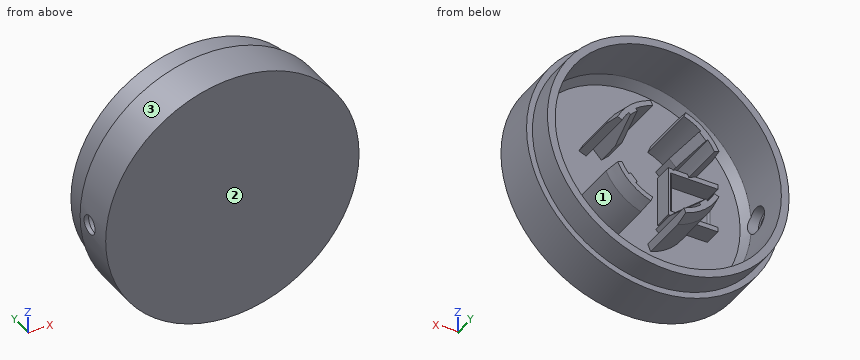
from build123d import *
from OCP.BRepFilletAPI import BRepFilletAPI_MakeChamfer

# Parameters (mm, degrees)
EXTRUDE_1_DEPTH     = 7
OTHER_START         = -47.7
OTHER_1_OUTLINE_R   = 5.1
OTHER_1_DEPTH       = 35.8
OTHER_START_2       = -30.461492928
OTHER_1_2_DEPTH     = 18.561492928
OTHER_START_3       = -51
OTHER_1_3_OUTLINE_R = 3.65
OTHER_1_3_DEPTH     = 3.3
OTHER_START_4       = 2
OTHER_1_4_DEPTH     = 1
OTHER_START_5       = 2.8
OTHER_1_5_DEPTH     = 7.2
OTHER_START_6       = -3
OTHER_1_6_DEPTH     = 0.709959236
EXTRUDE_2_DEPTH     = 24
EXTRUDE_2_2_DEPTH   = 24
EXTRUDE_2_3_DEPTH   = 24
EXTRUDE_2_4_DEPTH   = 24
CHAMFER_1_SIZE      = 6
CHAMFER_1_SIZE2     = 1.057961884
CHAMFER_2_SIZE      = 6
CHAMFER_2_SIZE2     = 1.057961884
CHAMFER_3_SIZE      = 6
CHAMFER_3_SIZE2     = 1.057961884
CHAMFER_4_SIZE      = 6
CHAMFER_4_SIZE2     = 1.057961884
CHAMFER_5_SIZE      = 1.1
EXTRUDE_3_DEPTH     = 24
CHAMFER_6_SIZE      = 15
CHAMFER_6_SIZE2     = 4.019237886


with BuildPart() as part:
    # Sketch 1 → Revolve 1 (revolve)
    with BuildSketch(Plane.XY):
        Polygon((0, 0), (-49.5, 0), (-49.5, 17), (-47.2, 17), (-47.2, 27), (-44.2, 27), (-44.2, 7), (-42.2, 3), (0, 3), align=None)
    revolve(axis=Axis((0, 3, 0), (0, -1, 0)))

    # Sketch 2 → Extrude 1 (add)
    with BuildSketch(Plane(origin=(0, 3, 0), x_dir=(1, 0, 0), z_dir=(0, 1, 0))):
        Polygon((-10, -9.82), (-10, 9.82), (-29.4, 9.82), (-29.4, 7.82), (-12, 7.82), (-12, -7.82), (-29.4, -7.82), (-29.4, -9.82), align=None)
    extrude(amount=EXTRUDE_1_DEPTH)

    # Other 1: read off the stored shape, not the designer's step
    # Other 1 outline → Other 1 (cut)
    with BuildSketch(Plane.YZ.offset(OTHER_START)):
        with Locations((10.72, 0)):
            Circle(OTHER_1_OUTLINE_R)
    extrude(amount=OTHER_1_DEPTH, mode=Mode.SUBTRACT)

    # Other 1 2 outline → Other 1 2 (cut)
    with BuildSketch(Plane.YZ.offset(OTHER_START_2)):
        with BuildLine():
            Line((2.8, 7.92), (2.8, -7.92))
            Line((2.8, -7.92), (10, -7.92))
            Line((10, -7.92), (10, -5.048920677))
            ThreePointArc((10, -5.048920677), (5.62, 0), (10, 5.048920677))
            Line((10, 5.048920677), (10, 7.92))
            Line((10, 7.92), (2.8, 7.92))
        make_face()
    extrude(amount=OTHER_1_2_DEPTH, mode=Mode.SUBTRACT)

    # Other 1 3 outline → Other 1 3 (cut)
    with BuildSketch(Plane.YZ.offset(OTHER_START_3)):
        with Locations((10.72, 0)):
            Circle(OTHER_1_3_OUTLINE_R)
    extrude(amount=OTHER_1_3_DEPTH, mode=Mode.SUBTRACT)

    # Other 1 4 outline → Other 1 4 (add)
    with BuildSketch(Plane(origin=(0, 0, 0), x_dir=(1, 0, 0), z_dir=(0, 1, 0)).offset(OTHER_START_4)):
        Polygon((-30.461492928, -7.72), (-30.461492928, -7.92), (-29.317348784, -7.92), align=None)
        Polygon((-30.461492928, 7.92), (-30.461492928, 7.72), (-29.317348784, 7.92), align=None)
    extrude(amount=OTHER_1_4_DEPTH)

    # Other 1 5 outline → Other 1 5 (add)
    with BuildSketch(Plane(origin=(0, 0, 0), x_dir=(1, 0, 0), z_dir=(0, 1, 0)).offset(OTHER_START_5)):
        Polygon((-29.317348784, -7.92), (-29.4, -7.905552307), (-29.4, -7.92), align=None)
        Polygon((-29.4, 7.92), (-29.4, 7.905552307), (-29.317348784, 7.92), align=None)
    extrude(amount=OTHER_1_5_DEPTH)

    # Other 1 6 outline → Other 1 6 (add)
    with BuildSketch(Plane(origin=(0, 0, 0), x_dir=(0.9850633751005737, -0.17219218052939098, 0), z_dir=(0.17219218052939098, 0.9850633751005737, 0)).offset(OTHER_START_6)):
        Polygon((-29.361584648, 7.92), (-30.523077576, 7.72), (-30.523077576, -7.72), (-29.361584648, -7.92), align=None)
    extrude(amount=OTHER_1_6_DEPTH)

    # Chamfer 5
    chamfer_5_edges = [part.edges().sort_by_distance(p)[0] for p in [
        (-11.9, 10, 0),
    ]]
    chamfer(chamfer_5_edges, length=CHAMFER_5_SIZE)



with BuildPart() as body_2:
    # Sketch 4 → Extrude 2 (new body)
    with BuildSketch(Plane(origin=(0, 3, 0), x_dir=(1, 0, 0), z_dir=(0, 1, 0))):
        with BuildLine():
            Line((-18.006273941, 8.704831921), (-20.798259543, 9.82))
            ThreePointArc((-20.798259543, 9.82), (-15.239680095, 17.226495598), (-7.210659701, 21.84047588))
            Line((-7.210659701, 21.84047588), (-6.095491622, 19.048490278))
            ThreePointArc((-6.095491622, 19.048490278), (-13.113793992, 15.100609496), (-18.006273941, 8.704831921))
        make_face()
    extrude(amount=EXTRUDE_2_DEPTH)

    # Chamfer 4
    chamfer_4_edges = [body_2.edges().sort_by_distance(p)[0] for p in [
        (-15.239680095, 27, -17.226495598),
    ]]
    chamfer_4_side = [body_2.faces().sort_by_distance(p)[0] for p in [
        (-15.239680095, 15, -17.226495598),
    ]]
    chamfer(chamfer_4_edges, length=CHAMFER_4_SIZE, length2=CHAMFER_4_SIZE2, reference=chamfer_4_side[0])


with BuildPart() as body_3:
    # Sketch 4 → Extrude 2 2 (new body)
    with BuildSketch(Plane(origin=(0, 3, 0), x_dir=(1, 0, 0), z_dir=(0, 1, 0))):
        with BuildLine():
            Line((-18.006273941, -8.704831921), (-20.798259543, -9.82))
            ThreePointArc((-20.798259543, -9.82), (-15.239680095, -17.226495598), (-7.210659701, -21.84047588))
            Line((-7.210659701, -21.84047588), (-6.095491622, -19.048490278))
            ThreePointArc((-6.095491622, -19.048490278), (-13.113793992, -15.100609496), (-18.006273941, -8.704831921))
        make_face()
    extrude(amount=EXTRUDE_2_2_DEPTH)

    # Chamfer 1
    chamfer_1_edges = [body_3.edges().sort_by_distance(p)[0] for p in [
        (-15.239680095, 27, 17.226495598),
    ]]
    chamfer_1_side = [body_3.faces().sort_by_distance(p)[0] for p in [
        (-15.239680095, 15, 17.226495598),
    ]]
    chamfer(chamfer_1_edges, length=CHAMFER_1_SIZE, length2=CHAMFER_1_SIZE2, reference=chamfer_1_side[0])


with BuildPart() as body_4:
    # Sketch 4 → Extrude 2 3 (new body)
    with BuildSketch(Plane(origin=(0, 3, 0), x_dir=(1, 0, 0), z_dir=(0, 1, 0))):
        with BuildLine():
            Line((6.095491622, 19.048490278), (7.210659701, 21.84047588))
            ThreePointArc((7.210659701, 21.84047588), (15.239680095, 17.226495598), (20.798259543, 9.82))
            Line((20.798259543, 9.82), (18.006273941, 8.704831921))
            ThreePointArc((18.006273941, 8.704831921), (13.113793992, 15.100609496), (6.095491622, 19.048490278))
        make_face()
    extrude(amount=EXTRUDE_2_3_DEPTH)

    # Chamfer 3
    chamfer_3_edges = [body_4.edges().sort_by_distance(p)[0] for p in [
        (15.239680095, 27, -17.226495598),
    ]]
    chamfer_3_side = [body_4.faces().sort_by_distance(p)[0] for p in [
        (15.239680095, 15, -17.226495598),
    ]]
    chamfer(chamfer_3_edges, length=CHAMFER_3_SIZE, length2=CHAMFER_3_SIZE2, reference=chamfer_3_side[0])


with BuildPart() as body_5:
    # Sketch 4 → Extrude 2 4 (new body)
    with BuildSketch(Plane(origin=(0, 3, 0), x_dir=(1, 0, 0), z_dir=(0, 1, 0))):
        with BuildLine():
            Line((18.006273941, -8.704831921), (20.798259543, -9.82))
            ThreePointArc((20.798259543, -9.82), (15.239680095, -17.226495598), (7.210659701, -21.84047588))
            Line((7.210659701, -21.84047588), (6.095491622, -19.048490278))
            ThreePointArc((6.095491622, -19.048490278), (13.113793992, -15.100609496), (18.006273941, -8.704831921))
        make_face()
    extrude(amount=EXTRUDE_2_4_DEPTH)

    # Chamfer 2
    chamfer_2_edges = [body_5.edges().sort_by_distance(p)[0] for p in [
        (15.239680095, 27, 17.226495598),
    ]]
    chamfer_2_side = [body_5.faces().sort_by_distance(p)[0] for p in [
        (15.239680095, 15, 17.226495598),
    ]]
    chamfer(chamfer_2_edges, length=CHAMFER_2_SIZE, length2=CHAMFER_2_SIZE2, reference=chamfer_2_side[0])


with BuildPart() as part_1:
    add(part.part)

    add(body_2.part)  # Extrude 3 merges body 2

    add(body_3.part)  # Extrude 3 merges body 3

    add(body_4.part)  # Extrude 3 merges body 4

    add(body_5.part)  # Extrude 3 merges body 5
    # Sketch 5 → Extrude 3 (add)
    with BuildSketch(Plane(origin=(0, 3, 0), x_dir=(1, 0, 0), z_dir=(0, 1, 0))):
        with BuildLine():
            Line((-9.275848781, 11.832874951), (-12.730982797, 15.424722916))
            ThreePointArc((-12.730982797, 15.424722916), (-14.142135624, 14.142135624), (-15.424722916, 12.730982797))
            Line((-15.424722916, 12.730982797), (-12.02081528, 9.192388155))
            Line((-12.02081528, 9.192388155), (-9.275848781, 11.832874951))
        make_face()
        with BuildLine():
            ThreePointArc((15.424722916, 12.730982797), (14.142135624, 14.142135624), (12.730982797, 15.424722916))
            Line((12.730982797, 15.424722916), (9.192388155, 12.02081528))
            Line((9.192388155, 12.02081528), (11.832874951, 9.275848781))
            Line((11.832874951, 9.275848781), (15.424722916, 12.730982797))
        make_face()
        with BuildLine():
            ThreePointArc((12.730982797, -15.424722916), (14.142135624, -14.142135624), (15.424722916, -12.730982797))
            Line((15.424722916, -12.730982797), (12.02081528, -9.192388155))
            Line((12.02081528, -9.192388155), (9.275848781, -11.832874951))
            Line((9.275848781, -11.832874951), (12.730982797, -15.424722916))
        make_face()
        with BuildLine():
            ThreePointArc((-15.424722916, -12.730982797), (-14.142135624, -14.142135624), (-12.730982797, -15.424722916))
            Line((-12.730982797, -15.424722916), (-9.192388155, -12.02081528))
            Line((-9.192388155, -12.02081528), (-11.832874951, -9.275848781))
            Line((-11.832874951, -9.275848781), (-15.424722916, -12.730982797))
        make_face()
    extrude(amount=EXTRUDE_3_DEPTH)

    # Chamfer 6: one chamfer whose edges measure the first distance from different faces: ONE call of the kernel's chamfer builder (chamfer() names one face for all edges)
    chamfer_6_edges_1 = [part_1.edges().sort_by_distance(p)[0] for p in [
        (-10.648332031, 27, -10.512631553),
    ]]
    chamfer_6_side_1 = [part_1.faces().sort_by_distance(p)[0] for p in [
        (-10.570396404, 15.633162389, -10.587600771),
    ]]
    chamfer_6_edges_2 = [part_1.edges().sort_by_distance(p)[0] for p in [
        (10.512631553, 27, -10.648332031),
    ]]
    chamfer_6_side_2 = [part_1.faces().sort_by_distance(p)[0] for p in [
        (10.512631553, 15, -10.648332031),
    ]]
    chamfer_6_edges_3 = [part_1.edges().sort_by_distance(p)[0] for p in [
        (10.648332031, 27, 10.512631553),
    ]]
    chamfer_6_side_3 = [part_1.faces().sort_by_distance(p)[0] for p in [
        (10.648332031, 15, 10.512631553),
    ]]
    chamfer_6_edges_4 = [part_1.edges().sort_by_distance(p)[0] for p in [
        (-10.512631553, 27, 10.648332031),
    ]]
    chamfer_6_side_4 = [part_1.faces().sort_by_distance(p)[0] for p in [
        (-10.447673128, 15.521619556, 10.715860754),
    ]]
    chamfer_6 = BRepFilletAPI_MakeChamfer(part_1.part.solid().wrapped)
    for e in chamfer_6_edges_1:
        chamfer_6.Add(CHAMFER_6_SIZE, CHAMFER_6_SIZE2, e.wrapped, chamfer_6_side_1[0].wrapped)  # the first distance lies on this face
    for e in chamfer_6_edges_2:
        chamfer_6.Add(CHAMFER_6_SIZE, CHAMFER_6_SIZE2, e.wrapped, chamfer_6_side_2[0].wrapped)  # the first distance lies on this face
    for e in chamfer_6_edges_3:
        chamfer_6.Add(CHAMFER_6_SIZE, CHAMFER_6_SIZE2, e.wrapped, chamfer_6_side_3[0].wrapped)  # the first distance lies on this face
    for e in chamfer_6_edges_4:
        chamfer_6.Add(CHAMFER_6_SIZE, CHAMFER_6_SIZE2, e.wrapped, chamfer_6_side_4[0].wrapped)  # the first distance lies on this face
    add(Compound.cast(chamfer_6.Shape()), mode=Mode.REPLACE)


solid = part_1.part
Input: part model. Units: mm. Frame: model coordinates. Face numbers are marked on the shaded views. Coordinates: 2 decimals unless noted, no trailing zeros. Loops run counter-clockwise (first coordinate to the right, second up) from the corner with the lowest first, then second, coordinate; pieces in that order, holes last. Notation, with made-up numbers: (27.25, 63.25) -> (68.25, 63.25) arc R18 ccw to (68.25, 73.25) -> close; hole circle Ø5 at (6, -30). An arc over 180 degrees is marked (long way). Write item = value, one per line. Start each with the question number.
Item 1: Material intervals for line 1 (X direction, y = 15.75, z = 0); line 2 (Z direction, x = 20.5, y = 18.75); line 3 (Y direction, x = -48.5, z = 0), sorted ascending.
Item 2: Cut plane B-B, the plane y = 18.75. Count the separate pieces of the cut face and the enclosed holes in it, plus the area to 3 significant figures.
Item 3: First-contact query: P1, Ø1.1, axis at x = -11, y = 8, coming from the -Z side; P2, Ø10, axis at y = 6, z = 9, coming from the +X side; P3, Ø6, axis at y = 12, z = -15.5, coming from the +X side; P4, Ø10, axis at x = -11, z = -3.5, coming from the -Y side. Flat tips, straight axial feed; report the tip coordinate or a pass-through.
Item 4: Mould query, pull axis X, two halves, no side actions, for the marked faces 1, 2 and 3. Classes: pulls with the +X half, pulls with the -X half, needs draft (parallel to the pull), parting line crosses it, or undercut.
Item 5: Cut plane A-A, the plane z = 0. Return loops of the section in (x, y).
Ans:
q1.line_1 = -49.5 to -47.7, 44.2 to 49.5
q1.line_2 = -42.52 to -39.16, -10.43 to -9.7, 9.7 to 10.43, 39.16 to 42.52
q1.line_3 = 0 to 7.07, 14.37 to 17
q2.separate_pieces = 5
q2.enclosed_holes = 1
q2.area = 1,120 mm²
q3.P1 = -48.38
q3.P2 = 49.34
q3.P3 = 47.9
q3.P4 = 0
q4.face_1 = undercut
q4.face_2 = needs draft
q4.face_3 = parting line crosses it
q5.outline = (-49.5, 0) -> (49.5, 0) -> (49.5, 17) -> (47.2, 17) -> (47.2, 27) -> (44.2, 27) -> (44.2, 7) -> (42.2, 3) -> (-10, 3) -> (-10, 10) -> (-10.8, 10) -> (-11.9, 8.9) -> (-11.9, 2.8) -> (-29.32, 2.8) -> (-30.46, 3) -> (-42.2, 3) -> (-43.51, 5.62) -> (-47.7, 5.62) -> (-47.7, 7.07) -> (-49.5, 7.07) -> close; (-49.5, 14.37) -> (-47.7, 14.37) -> (-47.7, 15.82) -> (-44.2, 15.82) -> (-44.2, 27) -> (-47.2, 27) -> (-47.2, 17) -> (-49.5, 17) -> close
